```python
from build123d import *

# Parameters (mm, degrees)
BOSS_EXTRUDE1_DEPTH         = 19.05
F_1_4_20_TAPPED_HOLE1_D     = 5.1054
F_1_4_20_TAPPED_HOLE1_DEPTH = 16.51
F_1_4_20_TAPPED_HOLE1_TIP   = 1.533816902
SKETCH4_R                   = 6.35
CUT_EXTRUDE1_DEPTH          = 19.05


with BuildPart() as part:
    # Sketch1 → Boss-Extrude1 (new body)
    with BuildSketch(Plane.XY):
        with BuildLine():
            Line((-3.175, -28.575), (-3.175, -22.225))
            ThreePointArc((-3.175, -22.225), (0, -19.05), (3.175, -22.225))
            Line((3.175, -22.225), (3.175, -28.575))
            Line((3.175, -28.575), (9.525, -28.575))
            Line((9.525, -28.575), (9.525, 28.575))
            Line((9.525, 28.575), (3.175, 28.575))
            Line((3.175, 28.575), (3.175, 22.225))
            ThreePointArc((3.175, 22.225), (0, 19.05), (-3.175, 22.225))
            Line((-3.175, 22.225), (-3.175, 28.575))
            Line((-3.175, 28.575), (-9.525, 28.575))
            Line((-9.525, 28.575), (-9.525, -28.575))
            Line((-9.525, -28.575), (-3.175, -28.575))
        make_face()
    extrude(amount=BOSS_EXTRUDE1_DEPTH)

    # 1/4-20 Tapped Hole1
    with Locations(Plane.XY.offset(19.05)):
        with Locations((0, 12.7), (0, -12.7)):
            Hole(F_1_4_20_TAPPED_HOLE1_D / 2, depth=F_1_4_20_TAPPED_HOLE1_DEPTH)
            with Locations((0, 0, -(F_1_4_20_TAPPED_HOLE1_DEPTH + F_1_4_20_TAPPED_HOLE1_TIP / 2))):  # 118° drill point
                Cone(0, F_1_4_20_TAPPED_HOLE1_D / 2, F_1_4_20_TAPPED_HOLE1_TIP, mode=Mode.SUBTRACT)

    # Sketch4 → Cut-Extrude1 (cut)
    with BuildSketch(Plane(origin=(9.525, 0, 0), x_dir=(0, 0, -1), z_dir=(1, 0, 0))):
        with Locations((-19.05, 0)):
            Circle(SKETCH4_R)
    extrude(amount=-CUT_EXTRUDE1_DEPTH, mode=Mode.SUBTRACT)


solid = part.part
```
Check sheet for the modelled part. Datum: model origin and axes. Units: mm. A direction names the side the tool comes from. Coordinates: 2 decimals unless noted, no trailing zeros. Loops run counter-clockwise (first coordinate to the right, second up) from the corner with the lowest first, then second, coordinate; pieces in that order, holes last. Notation, with made-up numbers: M 64.5,-12.5 L 83.5,-12.5 A25 ccw 83.5,0.5 Z; hole C 78,29 d7. An arc over 180 degrees is marked long. Answer as a JSON object with one key per item and string values.
1. Scan lines: L1, parallel to Y at x = 0, z = 7; L2, parallel to X at y = -26, z = 1 (3 decimals); L3, parallel to Y at x = -1, z = 13.5. Record each from-to range of solid material in increasing order. Write a range as from..to.
Outcome:
{"L1": "-19.05..-15.25, -10.15..10.15, 15.25..19.05", "L2": "-9.525..-3.175, 3.175..9.525", "L3": "-19.21..-15.05, -10.35..-3.09, 3.09..10.35, 15.05..19.21"}
2. Release check for a two-part mould opening along X. For faces 1 (the flat face through (3.175, 25, 9)), 2 (the flat face through (-6, 28.575, 9)), 3 (the flat face through (9.525, 0, 9)) record: pulls with the +X half, pulls with the -X half, needs draft (parallel to the pull), parting line crosses it, or undercut.
Outcome:
{"face 1": "undercut", "face 2": "needs draft", "face 3": "pulls with the +X half"}
3. Sectioned sample at B-B on y = 23. Record the cut outline in (x, z) (3 decimals), and give its area (3 significant figures).
Outcome:
{"outline": "M -9.525,0 L -3.175,0 L -3.175,19.05 L -9.525,19.05 Z; M 3.175,0 L 9.525,0 L 9.525,19.05 L 3.175,19.05 Z", "area": "242 mm²"}
4. Depth check by flat-ended pin: P1, Ø6.5, axis at x = 0, y = -12.7, coming from the -Z side; P2, Ø1, axis at x = 2, z = 13.5, coming from the +Y side; P3, Ø1, axis at x = 1, z = 10.5, coming from the -Y side. Enter the tip coordinate at first touch or a pass-through.
Outcome:
{"P1": "z = 0", "P2": "y = 20.27", "P3": "y = -19.43"}
5. Sectioned sample at A-A on z = 10.75. Record the cut outline in (x, y) (3 decimals), and give its area (3 significant figures).
Outcome:
{"outline": "M -9.525,-28.575 L -3.175,-28.575 L -3.175,-22.225 A3.175 cw 3.175,-22.225 L 3.175,-28.575 L 9.525,-28.575 L 9.525,28.575 L 3.175,28.575 L 3.175,22.225 A3.175 cw -3.175,22.225 L -3.175,28.575 L -9.525,28.575 Z; hole C 0,-12.7 d5.105; hole C 0,12.7 d5.105", "area": "935 mm²"}
6. Sectioned sample at D-D on x = -5.25. Record the cut outline in (y, z) (3 decimals).
Outcome:
{"outline": "M -28.575,0 L 28.575,0 L 28.575,19.05 L 6.35,19.05 A6.35 cw -6.35,19.05 L -28.575,19.05 Z"}
7. Access from +Z, -Z, +X, -X, +Y, -Y to the whole of each face (thin tool, end or side, straight path). Record for faces 4 (the flat face through (0, -17, 19.05)), 5 (the flat face through (3.175, -25, 9)), 6 (the flat face through (-3.175, 25, 9)), 7 (the cylindrical face through (0.553, -15.192, 10.679)), 8 (the flat face through (-6, -28.575, 9)).
Outcome:
{"face 4": "+Z, +X, -X, +Y, -Y", "face 5": "+Z, -Z, -Y", "face 6": "+Z, -Z, +Y", "face 7": "+Z", "face 8": "+Z, -Z, +X, -X, -Y"}
8. Sectioned sample at C-C on z = 17.5. Record the cut outline in (x, y) (3 decimals), and give its area (3 significant figures).
Outcome:
{"outline": "M -9.525,-28.575 L -3.175,-28.575 L -3.175,-22.225 A3.175 cw 3.175,-22.225 L 3.175,-28.575 L 9.525,-28.575 L 9.525,-6.158 L -9.525,-6.158 Z; M -9.525,6.158 L 9.525,6.158 L 9.525,28.575 L 3.175,28.575 L 3.175,22.225 A3.175 cw -3.175,22.225 L -3.175,28.575 L -9.525,28.575 Z; hole C 0,-12.7 d5.105; hole C 0,12.7 d5.105", "area": "701 mm²"}
